Answer from the drawing. Dimensions are ordinates in mm from the lowest x, y and z of the part. A direction names the side the tool comes from. Round coordinates to 2 decimals unless told otherwise and drop trailing zeros. Write each loop counter-clockwise with the first axis right and the second up, starting at its lowest first coordinate (ties: lowest second). Pieces come first, ordered by that corner, then holes. Notation, with made-up numbers: (87.5, -14.75) - (115.5, -14.75) arc R22 ccw to (115.5, -0.75) - close; hole circle Ø5 at (-25, -20.75). An arc over 180 degrees is marked (long way). Write item = value, one per line. Start each with the question number.
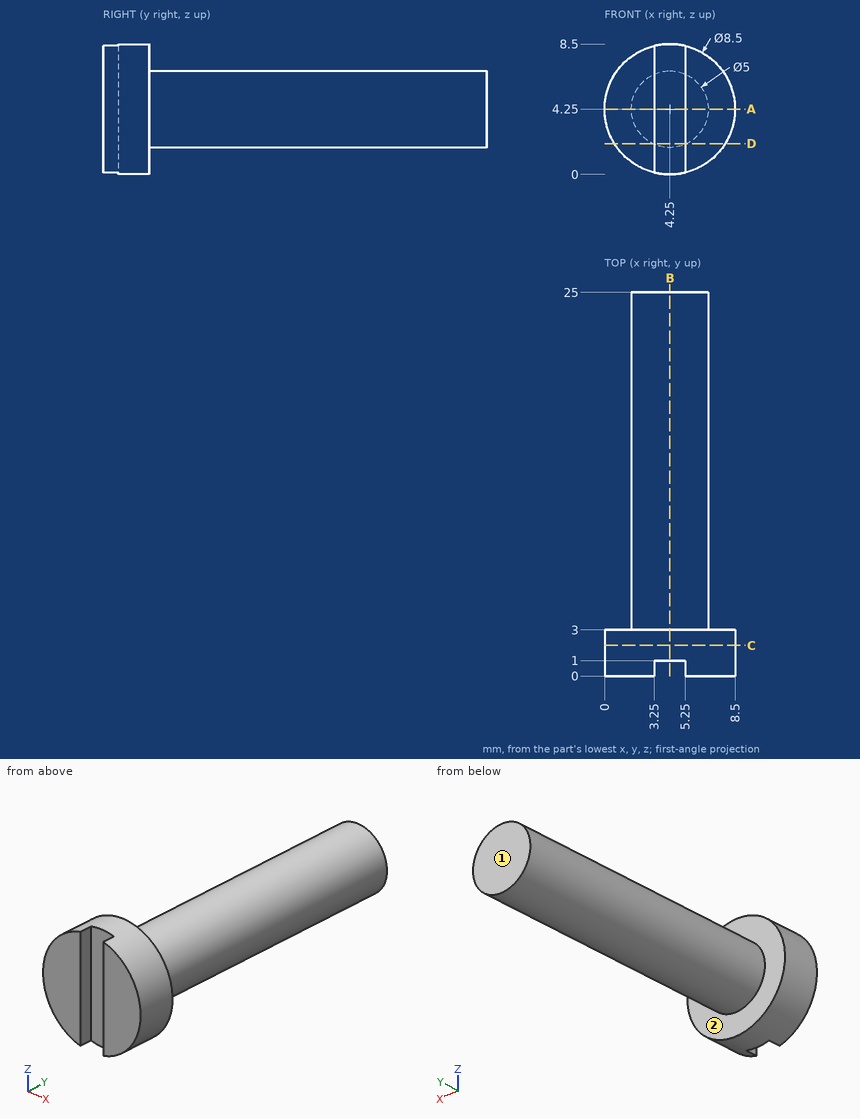
1. Find section D-D on z = 2. Give the vertices of the cut face in (x, y).
2. Find section A-A on z = 4.25. Give the vertices of the cut face in (x, y), plus the area to 4 significant figures.
3. Which of the six approach directions +Z, -Z, +X, -X, +Y, -Y give full straight-line access (tool end or side, diameter ignored) to the marked faces 1 and 2?
4. Each of these flat-tipped pins is pushed along its axis until it touches: pin 1 (5 mm diameter, centred on y = 12, z = 2.5, fed in from +X); pin 2 (1 mm diameter, centred on x = 1, y = 6.5, fed in from -Z); pin 3 (2 mm diameter, centred on x = 7.5, y = 12, fed in from +Z). Where does it stop, or does it pass through?
5. Find section C-C on y = 2. Give the vertices of the cut face in (x, z).
6. Find section B-B on x = 4.25. Give the vertices of the cut face in (y, z), plus the area to 3 significant figures.
7. Consider line 1 (X direction, y = 22.5, z = 4.25); line 2 (Y direction, x = 6, z = 6.5); line 3 (Y direction, x = 4.5, z = 4). Determine where each line is inside the solid, lowest interval first.
Answer key:
q1.outline = (0.64, 0) - (3.25, 0) - (3.25, 1) - (5.25, 1) - (5.25, 0) - (7.86, 0) - (7.86, 3) - (5.34, 3) - (5.34, 25) - (3.16, 25) - (3.16, 3) - (0.64, 3) - close
q2.outline = (0, 0) - (3.25, 0) - (3.25, 1) - (5.25, 1) - (5.25, 0) - (8.5, 0) - (8.5, 3) - (6.75, 3) - (6.75, 25) - (1.75, 25) - (1.75, 3) - (0, 3) - close
q2.area = 133.5 mm²
q3.face_1 = +Z, -Z, +X, -X, +Y
q3.face_2 = +Y
q4.pin_1 = 6.75
q4.pin_2 = through
q4.pin_3 = 5.34
q5.outline = circle Ø8.5 at (4.25, 4.25)
q6.outline = (1, 0) - (3, 0) - (3, 1.75) - (25, 1.75) - (25, 6.75) - (3, 6.75) - (3, 8.5) - (1, 8.5) - close
q6.area = 127 mm²
q7.line_1 = 1.75 to 6.75
q7.line_2 = 0 to 3
q7.line_3 = 1 to 25
